Source: CAD feature listing. Evaluate the final solid. Frame: model axes, mm. Face numbers are marked on the shaded views. A direction names the side the tool comes from. Give positions to 0.01 mm unless a question says otherwise; leave off trailing zeros. Loops run counter-clockwise (first coordinate to the right, second up) from the corner with the lowest first, then second, coordinate; pieces in that order, holes last. Notation, with made-up numbers: M 11,70 L 30,70 A29 ccw 30,92 Z; hole C 77.25,-2.5 d4. An arc over 180 degrees is marked long. Answer in a Markdown table with one row per item.
```python
from build123d import *

# Parameters (mm, degrees)
F0_W     = 18.995179
F0_H     = 18.995181
F1_DEPTH = 37.9984
F0_W_2   = 18.995181
F2_DEPTH = 18.9992


with BuildPart() as f1:
    # F0 (on Top) → F1 (new body)
    with BuildSketch(Plane.XY):
        with Locations((9.49759, 9.49759)):
            Rectangle(F0_W, F0_H)
    extrude(amount=-F1_DEPTH)

    # F0 (on Top) → F2 (join)
    with BuildSketch(Plane.XY):
        with Locations((-9.49759, -9.49759)):
            Rectangle(F0_W_2, F0_H)
        with Locations((-9.49759, 9.49759)):
            Rectangle(F0_W_2, F0_H)
        with Locations((9.49759, 9.49759)):
            Rectangle(F0_W, F0_H)
        with Locations((9.49759, -9.49759)):
            Rectangle(F0_W, F0_H)
    extrude(amount=-F2_DEPTH)


solid = f1.part
```
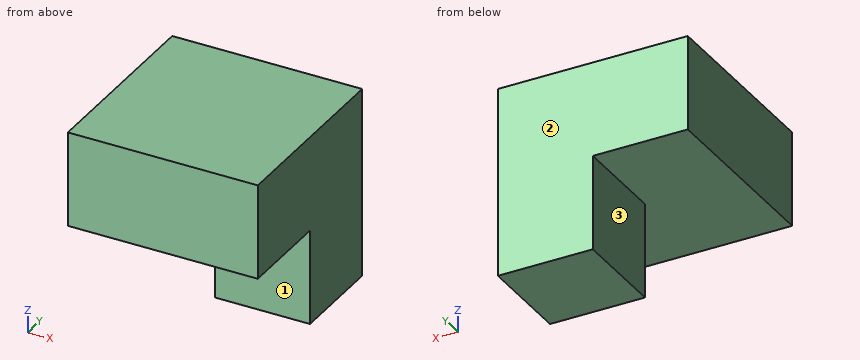
Q1. Contact query for flat-ended pins moving along their axis: pin 1 Ø5.5 at (y, z) = (6, -30) entering from -X; pin 2 Ø5.5 at (x, z) = (12.5, -28.5) entering from -Y; pin 3 Ø4 at (x, y) = (-9.5, 9) entering from -Z. Output: stop coordinate, or through.
Values follow:
| item | result |
|---|---|
| pin 1 | x = 0 |
| pin 2 | y = 0 |
| pin 3 | z = -19 |
Q2. Reachability of the marked faces 1, 2 and 3 from +Z, -Z, +X, -X, +Y, -Y: full face, straight path, thin tool, end or side. Return the list, or none.
Values follow:
| item | result |
|---|---|
| face 1 | -Z, +X, -X, -Y |
| face 2 | +Z, -Z, +X, -X, +Y |
| face 3 | -Z, -X, +Y, -Y |
Q3. Section query A-A (x = 16). Output: boundary loops of the cut face in (y, z).
Values follow:
| item | result |
|---|---|
| outline | M -19,-19 L 0,-19 L 0,-38 L 19,-38 L 19,0 L -19,0 Z |
Q4. Section query C-C (y = -11). Output: boundary loops of the cut face in (x, z), plus the area to 3 significant figures.
Values follow:
| item | result |
|---|---|
| outline | M -19,-19 L 19,-19 L 19,0 L -19,0 Z |
| area | 722 mm^2 |
Q5. Section query B-B (z = -31). Output: boundary loops of the cut face in (x, y).
Values follow:
| item | result |
|---|---|
| outline | M 0,0 L 19,0 L 19,19 L 0,19 Z |
Q6. Ray query, probe 1 along Y at (x, z) = (9, -32.5); probe 2 along Z at (x, y) = (14.5, -10.5). Return the intervals inside material, ascending. Write a range as from..to.
Values follow:
| item | result |
|---|---|
| probe 1 | 0..19 |
| probe 2 | -19..0 |
